from build123d import *

# Parameters (mm, degrees)
SKETCH1_R           = 2.1
BOSS_EXTRUDE1_DEPTH = 2.54
SKETCH2_W           = 47.761
SKETCH2_H           = 2.54
BOSS_EXTRUDE2_DEPTH = 25.4
FILLET1_R           = 2
FILLET2_R           = 1


with BuildPart() as part:
    # Sketch1 → Boss-Extrude1 (new body)
    with BuildSketch(Plane(origin=(0, 0, 0), x_dir=(1, 0, 0), z_dir=(0, 1, 0))):
        Polygon((-28.418010921, 1.935035563), (2.141991551, 1.935035563), (2.141991551, 29.143665766), (10.663279773, 29.143665766), (10.663279773, -3.055333898), (2.086284412, -3.055333898), (-28.52072334, -3.055333898), (-37.097720227, -3.055333898), (-37.097720227, 29.143665766), (-28.418010921, 29.143665766), align=None)
        with Locations(Location((-32.457720227, 24.503665766, 0), (0, 0, 270))):
            Circle(SKETCH1_R, mode=Mode.SUBTRACT)
        with Locations(Location((-32.457720227, 0.627665766, 0), (0, 0, 270))):
            Circle(SKETCH1_R, mode=Mode.SUBTRACT)
        with Locations(Location((6.023279773, 24.503665766, 0), (0, 0, 270))):
            Circle(SKETCH1_R, mode=Mode.SUBTRACT)
        with Locations(Location((6.023279773, 0.627665766, 0), (0, 0, 270))):
            Circle(SKETCH1_R, mode=Mode.SUBTRACT)
    extrude(amount=BOSS_EXTRUDE1_DEPTH)

    # Sketch2 → Boss-Extrude2 (add)
    with BuildSketch(Plane.XZ.offset(-2.54)):
        with Locations((-13.217220227, 4.325333898)):
            Rectangle(SKETCH2_W, SKETCH2_H)
    extrude(amount=BOSS_EXTRUDE2_DEPTH)

    # Fillet1
    fillet1_edges = [part.edges().sort_by_distance(p)[0] for p in [
        (2.141991551, 1.27, -29.143665766),
        (10.663279773, 1.27, -29.143665766),
        (-37.097720227, 1.27, -29.143665766),
        (-28.418010921, 1.27, -29.143665766),
        (-37.097720227, -22.86, 4.325333898),
        (10.663279773, -22.86, 4.325333898),
    ]]
    fillet(fillet1_edges, radius=FILLET1_R)

    # Fillet2
    fillet2_edges = [part.edges().sort_by_distance(p)[0] for p in [
        (10.663279773, 0, -12.044165934),
        (-28.418010921, 0, -14.539350664),
        (10.663279773, 2.54, -10.774165934),
        (-28.418010921, 2.54, -14.539350664),
        (-32.757865574, 0, -29.143665766),
        (-32.757865574, 2.54, -29.143665766),
        (2.141991551, 0, -14.539350664),
        (6.402635662, 0, -29.143665766),
        (-37.097720227, 0, -12.044165934),
        (10.077493335, 0, -28.557879329),
        (2.727777988, 0, -28.557879329),
        (-36.511933789, 0, -28.557879329),
        (-29.003797359, 0, -28.557879329),
        (-37.097720227, 2.54, -10.774165934),
        (6.402635662, 2.54, -29.143665766),
        (2.141991551, 2.54, -14.539350664),
        (10.077493335, 2.54, -28.557879329),
        (2.727777988, 2.54, -28.557879329),
        (-36.511933789, 2.54, -28.557879329),
        (-29.003797359, 2.54, -28.557879329),
    ]]
    fillet(fillet2_edges, radius=FILLET2_R)


solid = part.part
Can you work these out from the model? Positions are in its coordinate system, mm. A direction names the side the tool comes from. Give positions to 0.01 mm unless a question says otherwise; leave off trailing zeros. Write each loop counter-clockwise with the first axis right and the second up, starting at its lowest first coordinate (ties: lowest second). Pieces come first, ordered by that corner, then holes. Notation, with made-up numbers: M -9,-12.5 L 49,-12.5 A15 ccw 49,7.5 Z; hole C 10.25,10 d6. An arc over 180 degrees is marked long. Answer in a Markdown table with one row per item. Add a question column.
Item 1: Imagine slicing it at D-D, the plane y = -19.5. Write out the boundary of the cut face in (x, z), plus the area to 3 significant figures.
Item 2: Imagine slicing it at C-C, the plane x = -18. Write out the boundary of the cut face in (y, z), plus the area to 3 significant figures.
Item 3: For pin 1 Ø3 at (y, z) = (-1, -6) entering from +X; pin 2 Ø2.5 at (x, z) = (6.02, -24.5) entering from +Y; pin 3 Ø6 at (x, y) = (-27.5, -11) entering from -Z; pin 4 Ø1.3 at (x, y) = (-12, 0.5) entering from -Z, each with a flat end and sliding along its axis, tell me the tip position at first contact or that it passes through.
Item 4: Imagine slicing it at B-B, the plane x = 7. Write out the boundary of the cut face in (y, z), plus the area to 3 significant figures.
Item 5: Please list where these lines run through material, in increasing order: L1, parallel to X at y = 1.25, z = -18.5; L2, parallel to Z at x = -17, y = -8; L3, parallel to Y at x = 8, z = 1.
Item 6: On a 3-axis mill with a long thin cutter (end or side, diameter ignored), from which of +Z, -Z, +X, -X, +Y, -Y can I reach the whole of each face in a straight line? I mean faces 4 (the flat face through (-13, 0, -1)), 5 (the cylindrical face through (2.44, 0.29, -14.72)), 6 (the cylindrical face through (2.44, 2.25, -14.36)). Say none if no direction works.
Item 7: We'd pull the mould along Z, two halves only. Please class faces 1 (the cylindrical face through (-36.527, -22.259, 4.343)), 2 (the flat face through (-14, -10, 5.595)), 3 (the cylindrical face through (-33.736, 1.252, -26.17)): released by +Z, released by -Z, zero draft, split by the parting line, or undercut.
Item 8: Imagine slicing it at A-A, the plane z = -21.5. Write out the boundary of the cut face in (x, y).
Evaluation:
| question | item | result |
|---|---|---|
| 1 | outline | M -37.1,3.06 L 10.66,3.06 L 10.66,5.6 L -37.1,5.6 Z |
| 1 | area | 121 mm² |
| 2 | outline | M -22.86,3.06 L 0,3.06 L 0,-1.94 L 2.54,-1.94 L 2.54,5.6 L -22.86,5.6 Z |
| 2 | area | 77.2 mm² |
| 3 | pin 1 | stops at x = 10.53 |
| 3 | pin 2 | passes through |
| 3 | pin 3 | stops at z = 3.06 |
| 3 | pin 4 | stops at z = -1.94 |
| 4 | outline | M -22.86,3.06 L 0,3.06 L 0,1.23 L 2.54,1.23 L 2.54,5.6 L -22.86,5.6 Z; M 0,-28.14 A1 ccw 1,-29.14 L 1.54,-29.14 A1 ccw 2.54,-28.14 L 2.54,-26.36 L 0,-26.36 Z; M 0,-22.64 L 2.54,-22.64 L 2.54,-2.49 L 0,-2.49 Z |
| 4 | area | 127 mm² |
| 5 | L1 | x = -37.1 to -28.42, 2.14 to 10.66 |
| 5 | L2 | z = 3.06 to 5.6 |
| 5 | L3 | y = 0 to 2.54 |
| 6 | face 4 | -Z, +X, -X, -Y |
| 6 | face 5 | -Z, -Y |
| 6 | face 6 | -Z, +Y |
| 7 | face 1 | zero draft |
| 7 | face 2 | released by +Z |
| 7 | face 3 | undercut |
| 8 | outline | M -37.1,1 A1 ccw -36.1,0 L -29.42,0 A1 ccw -28.42,1 L -28.42,1.54 A1 ccw -29.42,2.54 L -36.1,2.54 A1 ccw -37.1,1.54 Z; M 2.14,1 A1 ccw 3.14,0 L 9.66,0 A1 ccw 10.66,1 L 10.66,1.54 A1 ccw 9.66,2.54 L 3.14,2.54 A1 ccw 2.14,1.54 Z |
